from build123d import *

# Parameters (mm, degrees)
ESBO_O2_R                      = 2.75
CORPO_DEPTH                    = 5
RAIO_DE_AL_VIO_DE_TENS_O_R15_R = 15
CHAMFER1_SIZE                  = 20


with BuildPart() as part:
    # Esboço2 → Corpo (new body)
    with BuildSketch(Plane(origin=(0, 0, 0), x_dir=(0, 0, -1), z_dir=(1, 0, 0))):
        with BuildLine():
            Line((0, 49), (16.5, 66))
            Line((16.5, 66), (45.5, 66))
            Line((45.5, 66), (62, 49))
            Line((62, 49), (62, 0))
            Line((62, 0), (62, -4))
            Line((62, -4), (107, -4))
            Line((107, -4), (107, -32))
            Line((107, -32), (0, -32))
            Line((0, -32), (0, 0))
            Line((0, 0), (0, 21.5))
            Line((0, 21.5), (20.838799284, 21.5))
            ThreePointArc((20.838799284, 21.5), (47.5, 34.5), (20.838799284, 47.5))
            Line((20.838799284, 47.5), (0, 47.5))
            Line((0, 47.5), (0, 49))
        make_face()
        with Locations((48.5, 52)):
            Circle(ESBO_O2_R, mode=Mode.SUBTRACT)
        with Locations((13.5, 52)):
            Circle(ESBO_O2_R, mode=Mode.SUBTRACT)
        with Locations((48.5, 17)):
            Circle(ESBO_O2_R, mode=Mode.SUBTRACT)
        with Locations((13.5, 17)):
            Circle(ESBO_O2_R, mode=Mode.SUBTRACT)
        with BuildLine():
            Line((69, -15.5), (75, -15.5))
            ThreePointArc((75, -15.5), (77.5, -18), (75, -20.5))
            Line((75, -20.5), (69, -20.5))
            ThreePointArc((69, -20.5), (66.5, -18), (69, -15.5))
        make_face(mode=Mode.SUBTRACT)
        with BuildLine():
            Line((84, -15.5), (90, -15.5))
            ThreePointArc((90, -15.5), (92.5, -18), (90, -20.5))
            Line((90, -20.5), (84, -20.5))
            ThreePointArc((84, -20.5), (81.5, -18), (84, -15.5))
        make_face(mode=Mode.SUBTRACT)
    extrude(amount=-CORPO_DEPTH)

    # Raio de Alívio de Tensão - R15
    raio_de_al_vio_de_tens_o_r15_edges = [part.edges().sort_by_distance(p)[0] for p in [
        (-2.5, -4, -62),
    ]]
    fillet(raio_de_al_vio_de_tens_o_r15_edges, radius=RAIO_DE_AL_VIO_DE_TENS_O_R15_R)

    # Chamfer1
    chamfer1_edges = [part.edges().sort_by_distance(p)[0] for p in [
        (-2.5, -32, 0),
    ]]
    chamfer(chamfer1_edges, length=CHAMFER1_SIZE)


solid = part.part
The model under review builds one solid part; all positions refer to its coordinate system, in mm. A direction names the side the tool comes from. Round coordinates to 2 decimals unless told otherwise and drop trailing zeros. Write each loop counter-clockwise with the first axis right and the second up, starting at its lowest first coordinate (ties: lowest second). Pieces come first, ordered by that corner, then holes. Notation, with made-up numbers: (-11.5, -18.5) -> (42.5, -18.5) arc R25 ccw to (42.5, 15.5) -> close; hole circle Ø8 at (-25, 45.25). An arc over 180 degrees is marked (long way). Answer as a JSON object with one key per item and string values.
1. We need section A-A on z = -31. State the section outline as (x, y) points.
Results found:
{"outline": "(-5, -32) -> (0, -32) -> (0, 18) -> (-5, 18) -> close; (-5, 51) -> (0, 51) -> (0, 66) -> (-5, 66) -> close"}
2. We need section D-D on y = 34.5. State the section outline as (x, z) points.
Results found:
{"outline": "(-5, -62) -> (0, -62) -> (0, -47.5) -> (-5, -47.5) -> close"}
3. We need section B-B on x = -3.3. State the section outline as (y, z) points, and give its area (3 significant figures).
Results found:
{"outline": "(-32, -107) -> (-4, -107) -> (-4, -77) arc R15 cw to (11, -62) -> (49, -62) -> (66, -45.5) -> (66, -16.5) -> (49, 0) -> (47.5, 0) -> (47.5, -20.84) arc R16.5 cw (long way) to (21.5, -20.84) -> (21.5, 0) -> (-12, 0) -> (-32, -20) -> close; hole (-20.5, -90) arc R2.5 ccw to (-15.5, -90) -> (-15.5, -84) arc R2.5 ccw to (-20.5, -84) -> close; hole (-20.5, -75) arc R2.5 ccw to (-15.5, -75) -> (-15.5, -69) arc R2.5 ccw to (-20.5, -69) -> close; hole circle Ø5.5 at (17, -48.5); hole circle Ø5.5 at (17, -13.5); hole circle Ø5.5 at (52, -48.5); hole circle Ø5.5 at (52, -13.5)", "area": "5,430 mm^2"}
4. To check wall thickness, follow line 1 along Y through (x, z) = (-4.5, -88); line 2 along Y through (x, z) = (-1.3, -13.5); line 3 along Y through (x, z) = (-2.9, -48.5). State the ranges of each line that lie inside material, in increasing order.
Results found:
{"line 1": "y = -32 to -20.5, -15.5 to -4", "line 2": "y = -25.5 to 14.25, 19.75 to 21.5, 47.5 to 49.25, 54.75 to 62.91", "line 3": "y = -32 to 14.25, 19.75 to 49.25, 54.75 to 62.91"}
5. The part is to be moulded in two halves that separate along Y. For faces 6 (the face through (-2.465, 57.619, -53.634)), 7 (the face through (-2, -18, -107)), 8 (the face through (-2, 47.5, -11)), say which applies: pulls with the +Y half, pulls with the -Y half, needs draft (parallel to the pull), parting line crosses it, or undercut.
Results found:
{"face 6": "pulls with the +Y half", "face 7": "needs draft", "face 8": "undercut"}
6. We need section C-C on z = -13.5. State the section outline as (x, y) points, and give its area (3 significant figures).
Results found:
{"outline": "(-5, -25.5) -> (0, -25.5) -> (0, 14.25) -> (-5, 14.25) -> close; (-5, 19.75) -> (0, 19.75) -> (0, 21.5) -> (-5, 21.5) -> close; (-5, 47.5) -> (0, 47.5) -> (0, 49.25) -> (-5, 49.25) -> close; (-5, 54.75) -> (0, 54.75) -> (0, 62.91) -> (-5, 62.91) -> close", "area": "257 mm^2"}
7. Machinability: for faces 1 (the face through (-2, -4, -92)), 2 (the face through (0, 7, -42)), 3 (the face through (-2.5, -18.1, -66.5)), 4 (the face through (-2, 21.5, -10)), 5 (the face through (-2, -22, -10)), which of the approach directions +Z, -Z, +X, -X, +Y, -Y give a long, thin tool a straight path to every point of the face, cutting with its end or side? Answer none if there is none.
Results found:
{"face 1": "-Z, +X, -X, +Y", "face 2": "+Z, -Z, +X, +Y, -Y", "face 3": "+X, -X", "face 4": "+Z, +X, -X", "face 5": "+Z, +X, -X, -Y"}
8. Clearance check with flat-ended pins moving along their axes: pin 1 (2.5 mm diameter, centred on x = -2.5, z = -14, fed in from -Y); pin 2 (5 mm diameter, centred on y = 20.5, z = -24.5, fed in from -X); pin 3 (2.5 mm diameter, centred on x = -3, z = -73.5, fed in from +Y); pin 4 (1 mm diameter, centred on x = -4, z = -16, fed in from -Y). State where each tip first meets the part, or that it passes through.
Results found:
{"pin 1": "stops at y = -27.25", "pin 2": "stops at x = -5", "pin 3": "stops at y = -3.23", "pin 4": "stops at y = -28.5"}
